Solid Edge part; units mm, degrees
sketch "Sketch1" plane through (0, 0, 0) normal (1, 0, 0) x (0, 1, 0)
  line L0 (-30, -10) -> (30, -10)
  line L1 (30, -10) -> (30, 10)
  line L2 (30, 10) -> (-30, 10)
  line L3 (-30, 10) -> (-30, -10)
extrude "Protrusion1" add sketch "Sketch1" along normal blind 110
sketch "Sketch2" plane through (50, 0, 10) normal (0, 0, 1) x (1, 0, 0)
  circle A0 centre (25, 0) radius 22
extrude "ExtrudedCutout_1" cut sketch "Sketch2" against normal blind 30.1603
sketch "Sketch3" plane through (50, 0, 10) normal (0, 0, 1) x (1, 0, 0)
  circle A0 centre (25, 0) radius 26
extrude "ExtrudedCutout_2" cut sketch "Sketch3" against normal blind 2
sketch "Sketch4" plane through (0, 0, 0) normal (-1, 0, 0) x (0, -1, 0)
  line L0 (30, 10) -> (-30, 10)
  line L1 (-30, 10) -> (-30, -10)
  line L2 (-30, -10) -> (30, -10)
  line L3 (30, -10) -> (30, 10)
extrude "Cutout1" cut sketch "Sketch4" against normal blind 5
hole "Hole_2" at (5, 15, 0) direction (1, 0, 0) diameter 11 depth 37.3 tip angle 118
hole "Hole1" at (5, -15, 0) direction (1, 0, 0) diameter 11 depth 37.3 tip angle 118
properties material "Steel - Stainless:1.4301 , X5CrNi18-10"
The listing builds one solid part. Answer for the finished solid, in the listing's coordinates (mm). A direction names the side the tool comes from. Round coordinates to 2 decimals unless told otherwise and drop trailing zeros. Order: outer loops, then holes, each group sorted by start corner. A loop starts at its lowest first (then second) coordinate and runs counter-clockwise, first axis right, second up. Notation, with made-up numbers: (-13, -11.75) - (10, -11.75) arc R14 cw to (10, 4.25) - close; hole circle Ø11 at (17.5, 43.25). An arc over 180 degrees is marked (long way). Write item = value, one per line. Start each with the question number.
1) Section C-C, the plane y = 0 is taken. Write down the section's boundary in (x, z), plus the area to 3 significant figures.
2) Section A-A, the plane x = 75 is taken. Write down the section's boundary in (y, z).
3) Section B-B, the plane z = -7.25 is taken. Write down the section's boundary in (x, y).
4) Section D-D, the plane x = 17.5 is taken. Write down the section's boundary in (y, z).
5) Straight lines are drawn through the part: L1, parallel to Y at x = 30, z = -0.5; L2, parallel to Y at x = 34.5, z = -4.5; L3, parallel to Z at x = 30, y = 15. For each, find the intervals that lie inside material, in ascending order.
6) Given pin 1 (9 mm diameter, centred on y = 15, z = 0, fed in from -X), flat-ended and moving along its own axis, determine where the tip first touches the part or whether it passes through.
7) For a pull along Y with two mould halves and no side action, classify faces 1 (the flat face through (57, 30, 0)), 2 (the flat face through (57, -30, 0)), 3 (the flat face through (110, 0, 0)), 4 (the cylindrical face through (23.91, -9.63, -1.19)) as released by +Y, released by -Y, zero draft, split by the parting line, or undercut.
8) For faces 5 (the cylindrical face through (23.91, 20.37, -1.19)), 6 (the flat face through (56, 12, 8)), 7 (the flat face through (45, 0, 10)), determine the directions among +Z, -Z, +X, -X, +Y, -Y from which every point of the face is accessible in a straight line to the end or side of a thin tool.
Results list:
q1.outline = (5, -10) - (53, -10) - (53, 8) - (49, 8) - (49, 10) - (5, 10) - close; (97, -10) - (110, -10) - (110, 10) - (101, 10) - (101, 8) - (97, 8) - close
q1.area = 1,200 mm^2
q2.outline = (-30, -10) - (-22, -10) - (-22, 8) - (-26, 8) - (-26, 10) - (-30, 10) - close; (22, -10) - (30, -10) - (30, 10) - (26, 10) - (26, 8) - (22, 8) - close
q3.outline = (5, -30) - (110, -30) - (110, 30) - (5, 30) - close; hole circle Ø44 at (75, 0)
q4.outline = (-30, -10) - (30, -10) - (30, 10) - (-30, 10) - close; hole circle Ø11 at (-15, 0); hole circle Ø11 at (15, 0)
q5.L1 = -30 to -20.48, -9.52 to 9.52, 20.48 to 30
q5.L2 = -30 to -18.16, -11.84 to 11.84, 18.16 to 30
q5.L3 = -10 to -5.5, 5.5 to 10
q6.pin_1 = 42.9
q7.face_1 = released by +Y
q7.face_2 = released by -Y
q7.face_3 = zero draft
q7.face_4 = undercut
q8.face_5 = -X
q8.face_6 = +Z
q8.face_7 = +Z, +X, -X, +Y, -Y
